```python
from build123d import *

# Parameters (mm, degrees)
SKETCH_1_R          = 2
EXTRUDE_1_DEPTH     = 20
SKETCH_2_W          = 18
SKETCH_2_H          = 18
CUT_EXTRUDE_1_DEPTH = 170.907643096


with BuildPart() as part:
    # 草图1 → 凸台-拉伸1 (new body)
    with BuildSketch(Plane.XY):
        Polygon((-48.727120284, 63.847904192), (31.272879716, -74.716160413), (48.593387792, -64.716160413), (-31.406612208, 73.847904192), align=None)
        with Locations((-35.246358171, 60.498539287)):
            Circle(SKETCH_1_R, mode=Mode.SUBTRACT)
        with Locations((-30.246358171, 51.838285249)):
            Circle(SKETCH_1_R, mode=Mode.SUBTRACT)
        with Locations((-7.501863714, 12.528261216)):
            Circle(SKETCH_1_R, mode=Mode.SUBTRACT)
        with Locations((-0.037744838, -0.482835818)):
            Circle(SKETCH_1_R, mode=Mode.SUBTRACT)
        with Locations((7.426374037, -13.493932851)):
            Circle(SKETCH_1_R, mode=Mode.SUBTRACT)
        with Locations((29.933133754, -52.395652337)):
            Circle(SKETCH_1_R, mode=Mode.SUBTRACT)
        with Locations((34.933133754, -61.055906375)):
            Circle(SKETCH_1_R, mode=Mode.SUBTRACT)
    extrude(amount=EXTRUDE_1_DEPTH)

    # 草图2 → 切除-拉伸1 (cut, through all)
    with BuildSketch(Plane(origin=(-39.828733576, 68.985390154, 0), x_dir=(0.8660254037844417, 0.4999999999999949, 0), z_dir=(-0.4999999999999949, 0.8660254037844417, 0))):
        with Locations((-0.274971923, -10)):
            Rectangle(SKETCH_2_W, SKETCH_2_H)
    extrude(amount=-CUT_EXTRUDE_1_DEPTH, mode=Mode.SUBTRACT)


solid = part.part
```
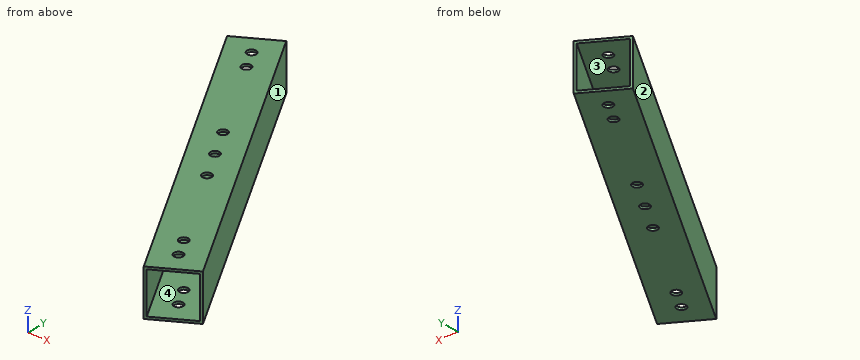
Work out the finished part from the listing and answer in its coordinate system (mm). Face numbers are marked on the shaded views. Round coordinates to 2 decimals unless told otherwise and drop trailing zeros. Write each loop counter-clockwise with the first axis right and the second up, starting at its lowest first coordinate (ties: lowest second). Pieces come first, ordered by that corner, then holes.
1) Flat-ended cylindrical pins translate along their axes: P1, Ø3.5, axis at x = 34.93, y = -61.06, coming from the +Z side; P2, Ø4, axis at y = -9, z = 13, coming from the -X side; P3, Ø5, axis at x = -0.04, y = -0.48, coming from the -Z side; P4, Ø12, axis at x = 36.5, z = 7, coming from the -Y side. Find the tip coordinate at first contact, or state that the pin passes through.
2) Determine the mould class of the marked faces 1, 2, 3 and 4 for opening direction X: pulls with the +X half, pulls with the -X half, needs draft (parallel to the pull), parting line crosses it, or undercut.
3) A cutting plane is placed at B-B on x = -7.5. Determine the outline of the cut face in (y, z).
4) A cutting plane is placed at C-C on y = 18.5. Determine the outline of the cut face in (x, z).
5) A cutting plane is placed at D-D on x = -20. Determine the outline of the cut face in (y, z).
6) A cutting plane is placed at A-A on z = 6. Determine the outline of the cut face in (x, y), and give its area (3 significant figures).
7) Consider probe 1 along Z at (x, y) = (28, -32); probe 2 along X at (y, z) = (-65, 16.5); probe 3 along X at (y, z) = (60, 18). Determine where each line is inside the solid, lowest interval first.
Entries:
1. P1: passes through
1. P2: stops at x = -7.82
1. P3: stops at z = 0
1. P4: stops at y = -74.72
2. face 1: pulls with the +X half
2. face 2: pulls with the -X half
2. face 3: undercut
2. face 4: undercut
3. outline: (-7.56, 0) - (10.53, 0) - (10.53, 1) - (-5.56, 1) - (-5.56, 19) - (10.53, 19) - (10.53, 20) - (-7.56, 20) - close; (14.53, 0) - (32.44, 0) - (32.44, 20) - (14.53, 20) - (14.53, 19) - (30.44, 19) - (30.44, 1) - (14.53, 1) - close
4. outline: (-22.55, 0) - (0.55, 0) - (0.55, 20) - (-22.55, 20) - close; hole (-21.39, 1) - (-0.61, 1) - (-0.61, 19) - (-21.39, 19) - close
5. outline: (14.09, 0) - (54.09, 0) - (54.09, 20) - (14.09, 20) - close; hole (16.09, 1) - (52.09, 1) - (52.09, 19) - (16.09, 19) - close
6. outline: (-48.73, 63.85) - (31.27, -74.72) - (32.14, -74.22) - (-47.86, 64.35) - close; (-32.27, 73.35) - (47.73, -65.22) - (48.59, -64.72) - (-31.41, 73.85) - close
6. area: 320 mm2
7. probe 1: z = 0 to 1, 19 to 20
7. probe 2: x = 25.66 to 26.82, 47.6 to 48.1
7. probe 3: x = -46.51 to -45.35, -24.57 to -23.41
